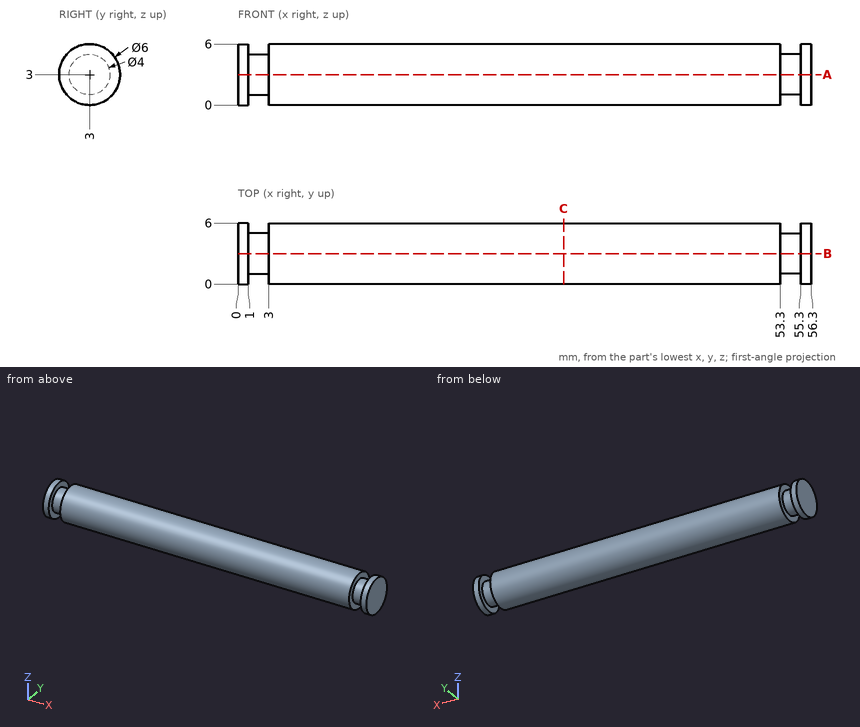
Geometry: see drawing. Coordinates: mm, zero at the bounding-box minimum. Coordinates: 2 decimals unless noted, no trailing zeros. Loops run counter-clockwise (first coordinate to the right, second up) from the corner with the lowest first, then second, coordinate; pieces in that order, holes last. Notation, with made-up numbers: M 23,84 L 78,84 A14 cw 78,99 Z; hole C 28.25,-6.5 d3. An arc over 180 degrees is marked long. Put each result on its own line as item: value. Start each with the question number.
1) Cut plane A-A on z = 3. Return the cut outline in (x, y), then the cut area to 3 significant figures.
2) Contact query for flat-ended pins moving along their axis: pin 1 Ø1 at (y, z) = (1.5, 1.5) entering from -X; pin 2 Ø1.5 at (x, y) = (10.5, 0.5) entering from +Z. Output: stop coordinate, or through.
3) Cut plane C-C on x = 32. Return the cut outline in (y, z), then the cut area to 3 significant figures.
4) Ray query, L1, parallel to X at y = 1.1, z = 1.15; L2, parallel to Z at x = 8, y = 2.9; L3, parallel to Z at x = 17, y = 4. Return the intervals inside material, ascending. Write a range as from..to.
The answers:
1. outline: M 0,0 L 1,0 L 1,1 L 3,1 L 3,0 L 53.3,0 L 53.3,1 L 55.3,1 L 55.3,0 L 56.3,0 L 56.3,6 L 55.3,6 L 55.3,5 L 53.3,5 L 53.3,6 L 3,6 L 3,5 L 1,5 L 1,6 L 0,6 Z
1. area: 330 mm²
2. pin 1: stops at x = 0
2. pin 2: stops at z = 5.44
3. outline: C 3,3 d6
3. area: 28.3 mm²
4. L1: x = 0..1, 3..53.3, 55.3..56.3
4. L2: z = 0..6
4. L3: z = 0.17..5.83
